```python
from build123d import *

# Parameters (mm, degrees)
F1_DEPTH = 50
F0_W     = 25
F0_H     = 50
F0_W_2   = 10
F0_H_2   = 40
F2_DEPTH = 75


with BuildPart() as f1:
    # F0 (on Top) → F1 (new body)
    with BuildSketch(Plane.XY):
        Polygon((27.5, 0), (-37.5, 0), (-37.5, -50), (-25, -50), (-25, -35), (2.5, -35), (2.5, -40), (27.5, -40), align=None)
    extrude(amount=F1_DEPTH)

    # F0 (on Top) → F2 (join)
    with BuildSketch(Plane.XY):
        with Locations((-50, -25)):
            Rectangle(F0_W, F0_H)
        with Locations((32.5, -20)):
            Rectangle(F0_W_2, F0_H_2)
        Polygon((57.5, 0), (37.5, 0), (37.5, -40), (37.5, -70), (57.5, -70), align=None)
    extrude(amount=F2_DEPTH)


solid = f1.part
```
The listing builds one solid part. Answer for the finished solid, in the listing's coordinates (mm). A direction names the side the tool comes from. Round coordinates to 2 decimals unless told otherwise and drop trailing zeros. Write each loop counter-clockwise with the first axis right and the second up, starting at its lowest first coordinate (ties: lowest second). Pieces come first, ordered by that corner, then holes. Notation, with made-up numbers: (66, 32) -> (103, 32) arc R23 cw to (103, 46) -> close; hole circle Ø2 at (72, 54.5). An arc over 180 degrees is marked (long way). Answer as a JSON object with one key per item and string values. Group by question number.
Q1. Section A-A (y = -48) is taken. Write down the section's boundary in (x, z).
Q2. Section D-D (y = -18.5) is taken. Write down the section's boundary in (x, z).
Q3. Which of the six approach directions +Z, -Z, +X, -X, +Y, -Y give full straight-line access (tool end or side, diameter ignored) to faces 4 (the face through (-44, -50, 37)), 5 (the face through (-37.5, -25, 62)), 6 (the face through (57.5, -35, 37)), 7 (the face through (46, -35, 75)), 8 (the face through (-11, -35, 25))?
Q4. Straight lines are drawn through the part: line 1 along X through (y, z) = (-44.5, 20.5); line 2 along X through (y, z) = (-22, 50.5); line 3 along Y through (x, z) = (-33.5, 13). For each, find the intervals that lie inside material, in ascending order.
Q5. Determine the mould class of faces 1 (the face through (-62.5, -25, 37)), 2 (the face through (47, -70, 37)), 3 (the face through (-5, -19, 50)) for opening direction X: pulls with the +X half, pulls with the -X half, needs draft (parallel to the pull), parting line crosses it, or undercut.
Q6. Section B-B (z = 55) is taken. Write down the section's boundary in (x, y).
Q7. Each of these flat-tipped pins is pushed along its axis until it touches: pin 1 Ø5 at (x, z) = (13, 16) entering from -Y; pin 2 Ø15 at (x, y) = (0, -13.5) entering from +Z. Where does it stop, or does it pass through?
Q8. Section C-C (z = 7) is taken. Write down the section's boundary in (x, y), plus the area to 3 significant figures.
Check values:
{
 "1": {"outline": "(-62.5, 0) -> (-25, 0) -> (-25, 50) -> (-37.5, 50) -> (-37.5, 75) -> (-62.5, 75) -> close; (37.5, 0) -> (57.5, 0) -> (57.5, 75) -> (37.5, 75) -> close"},
 "2": {"outline": "(-62.5, 0) -> (57.5, 0) -> (57.5, 75) -> (27.5, 75) -> (27.5, 50) -> (-37.5, 50) -> (-37.5, 75) -> (-62.5, 75) -> close"},
 "3": {"face 4": "+Z, -Z, -X, -Y", "face 5": "+Z, +Y, -Y", "face 6": "+Z, -Z, +X, +Y, -Y", "face 7": "+Z, +X, -X, +Y, -Y", "face 8": "+Z, -Z, -Y"},
 "4": {"line 1": "-62.5 to -25, 37.5 to 57.5", "line 2": "-62.5 to -37.5, 27.5 to 57.5", "line 3": "-50 to 0"},
 "5": {"face 1": "pulls with the -X half", "face 2": "needs draft", "face 3": "undercut"},
 "6": {"outline": "(-62.5, -50) -> (-37.5, -50) -> (-37.5, 0) -> (-62.5, 0) -> close; (27.5, -40) -> (37.5, -40) -> (37.5, -70) -> (57.5, -70) -> (57.5, 0) -> (27.5, 0) -> close"},
 "7": {"pin 1": "y = -40", "pin 2": "z = 50"},
 "8": {"outline": "(-62.5, -50) -> (-25, -50) -> (-25, -35) -> (2.5, -35) -> (2.5, -40) -> (37.5, -40) -> (37.5, -70) -> (57.5, -70) -> (57.5, 0) -> (-62.5, 0) -> close", "area": "5,640 mm^2"}
}
